Could you check a few things on this model? Use its own coordinates, in mm. Round coordinates to 2 decimals unless told otherwise and drop trailing zeros. Write each loop counter-clockwise with the first axis right and the second up, starting at its lowest first coordinate (ties: lowest second). Pieces come first, ordered by that corner, then holes. Notation, with made-up numbers: (60, -2.5) -> (106, -2.5) arc R35 cw to (106, 35.5) -> close; hole circle Ø4 at (41.25, 52.25). An arc over 180 degrees is marked (long way). Return JSON: item names as keys, results as strings.
from build123d import *

# Parameters (mm, degrees)
F1_DEPTH = 5.08


with BuildPart() as f1:
    # F0 (on Front) → F1 (new body)
    with BuildSketch(Plane.XZ):
        with BuildLine():
            Line((-78.91387, 129.106149), (-86.796143, 139.064049))
            ThreePointArc((-86.796143, 139.064049), (-95.286354, 143.796683), (-104.636317, 141.139675))
            ThreePointArc((-104.636317, 141.139675), (-109.36895, 132.649465), (-106.711943, 123.299502))
            Line((-106.711943, 123.299502), (-83.065122, 93.425803))
            ThreePointArc((-83.065122, 93.425803), (-74.574912, 88.693169), (-65.224949, 91.350177))
            Line((-65.224949, 91.350177), (64.227746, 193.819732))
            ThreePointArc((64.227746, 193.819732), (73.577709, 196.47674), (82.067919, 191.744106))
            Line((82.067919, 191.744106), (105.714739, 161.870408))
            ThreePointArc((105.714739, 161.870408), (108.371747, 152.520445), (103.639113, 144.030234))
            ThreePointArc((103.639113, 144.030234), (94.289151, 141.373227), (85.79894, 146.105861))
            Line((85.79894, 146.105861), (77.916667, 156.06376))
            Line((77.916667, 156.06376), (-107.305268, 9.449514))
            ThreePointArc((-107.305268, 9.449514), (-109.361582, 2.384159), (-103.364131, -1.879436))
            Line((-103.364131, -1.879436), (-45.04985, -1.879436))
            Line((-45.04985, -1.879436), (-45.04985, 10.820564))
            Line((-45.04985, 10.820564), (-41.87485, 10.820564))
            Line((-41.87485, 10.820564), (-41.87485, -1.879436))
            Line((-41.87485, -1.879436), (96.761584, -1.879436))
            Line((96.761584, -1.879436), (96.761584, 10.820564))
            Line((96.761584, 10.820564), (99.936584, 10.820564))
            Line((99.936584, 10.820564), (99.936584, -1.879436))
            Line((99.936584, -1.879436), (111.823284, -1.879436))
            ThreePointArc((111.823284, -1.879436), (133.252209, 5.274321), (142.385621, 25.937231))
            Line((142.385621, 25.937231), (142.385621, 105.471752))
            Line((142.385621, 105.471752), (129.685621, 105.471752))
            Line((129.685621, 105.471752), (129.685621, 108.646752))
            Line((129.685621, 108.646752), (142.385621, 108.646752))
            Line((142.385621, 108.646752), (142.385621, 246.527939))
            ThreePointArc((142.385621, 246.527939), (126.613941, 271.678994), (97.104619, 268.435318))
            Line((97.104619, 268.435318), (18.94209, 206.564998))
            Line((18.94209, 206.564998), (26.824363, 196.607098))
            Line((26.824363, 196.607098), (24.334888, 194.63653))
            Line((24.334888, 194.63653), (16.452615, 204.594429))
            Line((16.452615, 204.594429), (-78.91387, 129.106149))
        make_face()
    extrude(amount=F1_DEPTH)


solid = f1.part
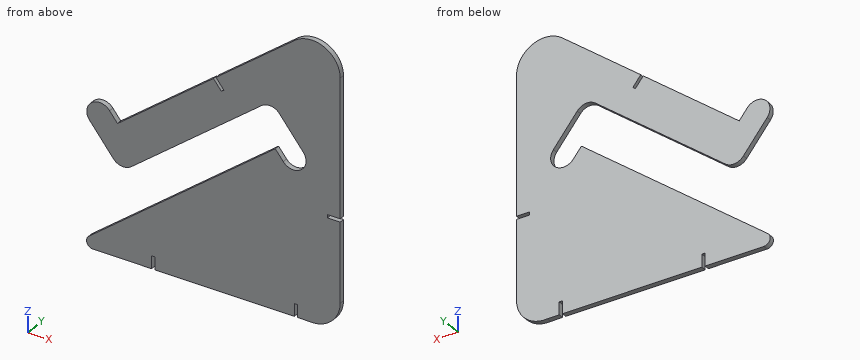
1) I want a section at D-D, the plane z = 76.5. Please give me the cut outline in (x, y).
Return value:
{"outline": "(-22.6, -5.08) -> (142.39, -5.08) -> (142.39, 0) -> (-22.6, 0) -> close"}
2) I want a section at A-A, the plane x = -91. Please give me the cut outline in (y, z).
Return value:
{"outline": "(-5.08, -1.88) -> (0, -1.88) -> (0, 22.36) -> (-5.08, 22.36) -> close; (-5.08, 103.45) -> (0, 103.45) -> (0, 142.5) -> (-5.08, 142.5) -> close"}
3) Will these pins go through, and if not, where does the flat tip stop? pin 1 Ø8 at (x, z) = (-54.5, 38.5) entering from +Y; pin 2 Ø2.5 at (x, y) = (136.5, -2) entering from -Z; pin 3 Ø1.5 at (x, y) = (107, -2.5) entering from -Z; pin 4 Ø1.5 at (x, y) = (138.5, -2) entering from +Z.
Return value:
{"pin 1": "y = 0", "pin 2": "z = 7.29", "pin 3": "z = -1.88", "pin 4": "z = 261.94"}
4) If I drill on probe 1 along Z at (x, y) = (23, -2.2); probe 2 along X at (y, z) = (-1.95, 139); probe 3 along X at (y, z) = (-3.05, 96), over which ranges is the centre line in solid material (lowest first)? Write a range as [from, to].
Return value:
{"probe 1": "[-1.88, 112.59], [161.19, 196.32], [201.44, 209.78]", "probe 2": "[-106.76, -86.75], [-66.41, -5.03], [56.36, 142.39]", "probe 3": "[-85.1, -59.35], [2.04, 142.39]"}
5) I want a section at B-B, the plane z = 165. Please give me the cut outline in (x, y), and give its area (3 significant figures).
Return value:
{"outline": "(-33.57, -5.08) -> (27.82, -5.08) -> (27.82, 0) -> (-33.57, 0) -> close; (103.24, -5.08) -> (142.39, -5.08) -> (142.39, 0) -> (103.24, 0) -> close", "area": "511 mm²"}
